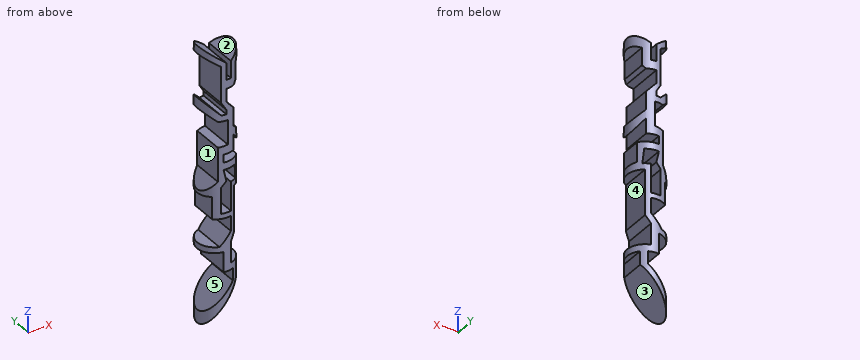
```python
from build123d import *

# Parameters (mm, degrees)
F0_R     = 10.675430612
F1_DEPTH = 137.16
F2_DEPTH = 38.1
F3_W     = 73.8532952964
F3_H     = 204.6351656318
F4_DEPTH = 12.7


with BuildPart() as f1:
    # F0 (on Top) → F1 (new body)
    with BuildSketch(Plane.XY):
        Circle(F0_R)
    extrude(amount=-F1_DEPTH)

    # F2 (add): a face of the model
    f2_faces = [f1.faces().sort_by_distance(p)[0] for p in [
        (0, 0, 0),
    ]]
    extrude(f2_faces, amount=F2_DEPTH)

    # F3 (on Front) → F4 (cut, symmetric)
    with BuildSketch(Plane.XZ):
        with Locations((0.4835147411, -55.2906431258)):
            Rectangle(F3_W, F3_H)
        Polygon((2.9173363, 19.1722828895), (11.8985436857, 25.6116390228), (15.7361086458, 21.5601604432), (6.9777617314, 16.1294173449), (6.9777617314, 5.8243007956), (5.2905785851, 3.9081033319), (0, 3.9081033319), (0, -3.7856895942), (5.2087670282, -9.4788996503), (5.2087670282, -20.1990260627), (15.5135185486, -30.6273752617), (12.1595710516, -34.4365797937), (5.1792738959, -25.212617591), (5.1792738959, -34.3119315803), (-1.5746362042, -34.3119315803), (-1.5746362042, -39.0876196325), (8.6516765878, -39.0876196325), (8.6516765878, -50.6781153381), (13.8188395649, -51.9570671022), (13.8188395649, -55.5720552802), (5.6630028412, -55.5720552802), (5.6630028412, -82.3548957705), (2.9173363, -87.0497524738), (2.9173363, -99.5368526672), (16.7356515435, -99.5368526672), (17.0829258859, -103.5451963544), (7.6496228576, -103.5451963544), (7.6496228576, -111.4576309919), (-13.9778433368, -140.0423496962), (-17.0550644398, -135.2102676343), (4.4348337688, -110.8033806086), (4.4348337688, -103.5782471299), (-1.5746362042, -103.5782471299), (-1.5746362042, -91.662183404), (-13.6558805862, -92.110427912), (-13.9778433368, -88.3942381419), (-3.6802912408, -88.3942381419), (2.9173363, -80.9010639787), (2.9173363, -71.9678923488), (-6.8503268994, -71.9678923488), (-6.8503268994, -58.7706156075), (-12.6116908069, -59.2697678805), (-4.392595496, -49.9350316823), (-4.392595496, -29.8299845308), (0.8731535636, -29.1371215135), (0.8731535636, -14.7255985066), (-4.392595496, -14.7255985066), (-13.9778433368, -6.2859314494), (-17.0550644398, -8.4015205503), (-13.7855187058, 0), (-2.8229181189, -11.0940886661), (0, -11.0940886661), (0, -8.4015205503), (-2.8229181189, -3.7856895942), (-2.8229181189, 17.5625272095), (-15.3241287917, 26.0248854756), (-17.0550644398, 32.3716513813), (0, 19.1722828895), (0, 9.1743338853), (2.9173363, 9.1743338853), align=None, mode=Mode.SUBTRACT)
        Polygon((6.0701598413, -43.3530472219), (-1.5746362042, -43.3530472219), (0, -50.2383581229), (-2.8229181189, -53.4444525838), (-2.8229181189, -68.9763724804), (2.9173363, -68.9763724804), (2.9173363, -51.8846450228), (6.8093192667, -51.8846450228), align=None)
    extrude(amount=F4_DEPTH, both=True, mode=Mode.SUBTRACT)


solid = f1.part
```
The model under review builds one solid part; all positions refer to its coordinate system, in mm. Face numbers are marked on the shaded views. A direction names the side the tool comes from. Round coordinates to 2 decimals unless told otherwise and drop trailing zeros. Write each loop counter-clockwise with the first axis right and the second up, starting at its lowest first coordinate (ties: lowest second). Pieces come first, ordered by that corner, then holes.
(1) Machinability: for the marked faces 4 and 5, which of the approach directions +Z, -Z, +X, -X, +Y, -Y give a long, thin tool a straight path to every point of the face, cutting with its end or side? Answer none if there is none.
(2) Wall thickness on L1, parallel to Z at x = 2.5, y = 9.25; L2, parallel to Z at x = -3.25, y = 0.75; L3, parallel to Z at x = -4, y = 6: over which ranges is each line inside the solid? List them lowest first.
(3) Mouldability with a two-part tool opening along Z and no side actions: class the marked faces 1, 2 and 3 as +Z half, -Z half, draft (parallel to the pull), parting line (faces both ways), or undercut.
(4) Insertion check: pin 1 (11.5 mm diameter, centred on y = -0.5, z = -23, fed in from -X); pin 2 (6 mm diameter, centred on y = 0, z = -44.5, fed in from -X); pin 3 (2.5 mm diameter, centred on y = -1.5, z = -108.5, fed in from +X). Each pin has a flat end and moves straight along its axis. Give the tip position at first contact, or say it passes through.
(5) We need section A-A on z = -41. Give the boundary of the cut face in (x, y).
Findings below:
1. face 4: +X, +Y, -Y
1. face 5: -X, +Y, -Y
2. L1: z = -118.26 to -113, -103.58 to -81.38, -71.97 to -68.98, -43.35 to -39.09, -34.31 to -6.52, 3.91 to 9.17
2. L2: z = -125.86 to -119.53, -91.72 to -87.91, -71.97 to -29.68, -14.73 to -10.66, 17.85 to 21.69
2. L3: z = -126.85 to -120.38, -91.75 to -88.39, -71.97 to -29.78, -14.73 to -9.9, 18.36 to 22.27
3. face 1: undercut
3. face 2: +Z half
3. face 3: -Z half
4. pin 1: stops at x = 0.87
4. pin 2: stops at x = -4.39
4. pin 3: stops at x = 7.65
5. outline: (-4.39, -9.73) arc R10.68 ccw to (8.65, -6.25) - (8.65, 6.25) arc R10.68 ccw to (-4.39, 9.73) - close
